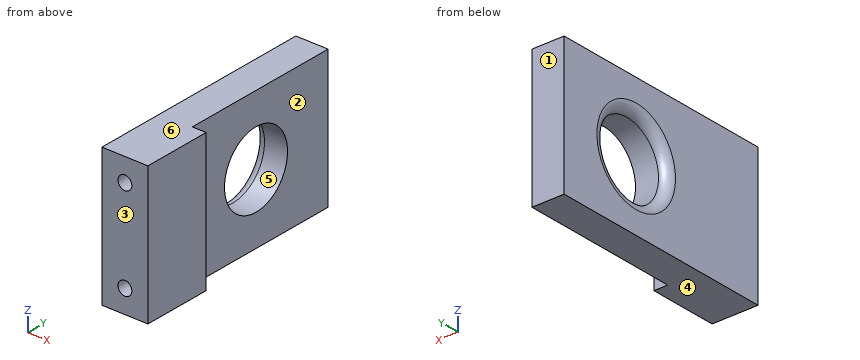
Autodesk Inventor part; units mm, degrees
ref_plane "YZ Plane" through (0, 0, 0) normal (1, 0, 0) x (0, 1, 0)
ref_plane "XZ Plane" through (0, 0, 0) normal (0, 1, 0) x (-1, 0, 0)
ref_plane "XY Plane" through (0, 0, 0) normal (0, 0, 1) x (1, 0, 0)
sketch "Sketch1" plane through (0, 0, 0) normal (0, 1, 0) x (-1, 0, 0)
  line L0 (0, 0) -> (10, 0)
  line L1 (10, 0) -> (10, -30)
  line L2 (10, -30) -> (0, -30)
  line L3 (0, -30) -> (0, 0)
  dimension "d0" = 10
  dimension "d1" = 30
extrude "Extrusion1" add sketch "Sketch1" along normal blind 50
sketch "Sketch2" plane through (0, 0, 0) normal (0, -1, 0) x (1, 0, 0)
  line L0 (0, 0) -> (0, -30)
  circle A0 centre (-5, -5) radius 1.5
  circle A1 centre (-5, -25) radius 1.5
  dimension "d7" = 3
extrude "Extrusion2" cut sketch "Sketch2" against normal blind 8
sketch "Sketch3" plane through (0, 0, 0) normal (1, 0, 0) x (0, 0, -1)
  line L0 (30, 0) -> (0, 0)
  circle A0 centre (15, 31.418) radius 8.125
  dimension "d11" = 16.25
extrude "Extrusion3" cut sketch "Sketch3" against normal up to surface (10 mm away)
fillet "Fillet1" radius 2 2 edges at (0, 31.418, -6.875) (-10, 31.418, -6.875)
sketch "Sketch5" plane through (0, 0, 0) normal (1, 0, 0) x (0, 0, -1)
  line L0 (30, 50) -> (0, 50)
  line L1 (30, 0) -> (30, 50)
  line L2 (0, 50) -> (30, 50)
  line L3 (30, 50) -> (30, 15)
  line L4 (30, 15) -> (0, 15)
  line L5 (0, 15) -> (0, 50)
  point P0 (0, 0)
  dimension "d15" = 35
extrude "Extrusion4" cut sketch "Sketch5" against normal blind 3
properties part number "Bracket_Support"
Read the model definition and answer for the solid it produces. Units are mm, in the model's axes. Face numbers are marked on the shaded views. A direction names the side the tool comes from. Round coordinates to 2 decimals unless told otherwise and drop trailing zeros. Write each loop counter-clockwise with the first axis right and the second up, starting at its lowest first coordinate (ties: lowest second). Pieces come first, ordered by that corner, then holes. Notation, with made-up numbers: (43, 7) - (93, 7) arc R9 ccw to (93, 24) - close; hole circle Ø4 at (13, -28.75). An arc over 180 degrees is marked (long way). One line per question, with ' | ' between items. Start each with the question number.
1. Section C-C (x = -5.25) is taken. Determine the outline of the cut face in (y, z) (3 decimals), and give its area (3 significant figures).
2. Section B-B (z = -1.75) is taken. Determine the outline of the cut face in (x, y), and give its area (3 significant figures).
3. Section D-D (x = -1.5) is taken. Determine the outline of the cut face in (y, z), and give its area (3 significant figures).
4. Find the intervals of material crossed by probe 1 along Y at (x, z) = (-4.45, -15); probe 2 along X at (y, z) = (23, -23.75); probe 3 along Y at (x, z) = (-0.25, -12.25), in increasing order. Write a range as [from, to].
5. For the marked faces 1 and 2, determine the directions among +Z, -Z, +X, -X, +Y, -Y from which every point of the face is accessible in a straight line to the end or side of a thin tool.
6. Each of these flat-tipped pins is pushed along its axis until it touches: pin 1 (2.5 mm diameter, centred on x = -1, z = -19, fed in from +Y); pin 2 (9 mm diameter, centred on y = 33.5, z = -10, fed in from +X); pin 3 (1.5 mm diameter, centred on x = -5, z = -24.5, fed in from -Y). Where does it stop, or does it pass through?
7. For a pull along Z with two mould halves and no side action, classify the marked faces 3, 4, 5 and 6 as +Z half, -Z half, draft (parallel to the pull), parting line (faces both ways), or undercut.
8. Section A-A (z = -15) is taken. Determine the outline of the cut face in (x, y), and give its area (3 significant figures).
Filled in:
1) outline: (0, -30) - (50, -30) - (50, 0) - (0, 0) - (0, -3.521) - (8, -3.521) - (8, -6.479) - (0, -6.479) - (0, -23.521) - (8, -23.521) - (8, -26.479) - (0, -26.479) - close; hole circle Ø16.25 at (31.418, -15) | area: 1,250 mm²
2) outline: (-10, 0) - (0, 0) - (0, 15) - (-3, 15) - (-3, 50) - (-10, 50) - close | area: 395 mm²
3) outline: (0, -30) - (15, -30) - (15, 0) - (0, 0) - close | area: 450 mm²
4) probe 1: [0, 23.29], [39.54, 50] | probe 2: [-10, -3] | probe 3: [0, 15]
5) face 1: +Z, -Z, +X, -X, +Y | face 2: +Z, -Z, +X, +Y
6) pin 1: y = 15 | pin 2: x = -3 | pin 3: y = 8
7) face 3: draft | face 4: -Z half | face 5: undercut | face 6: +Z half
8) outline: (-10, 0) - (0, 0) - (0, 15) - (-3, 15) - (-3, 23.29) - (-8, 23.29) arc R2 ccw to (-10, 21.29) - close; (-10, 41.54) arc R2 ccw to (-8, 39.54) - (-3, 39.54) - (-3, 50) - (-10, 50) - close | area: 280 mm²
